Verification items for this drawing (mm, ordinates from the low corner). A direction names the side the tool comes from. Give positions to 0.01 mm unless a question says otherwise; leave off trailing zeros. Loops run counter-clockwise (first coordinate to the right, second up) from the corner with the lowest first, then second, coordinate; pieces in that order, holes last. Notation, with made-up numbers: M -33.5,17 L -1.5,17 A12 cw -1.5,31 Z; hole C 84,-2 d7. An arc over 180 degrees is marked long. Use a Markdown table: item, result.
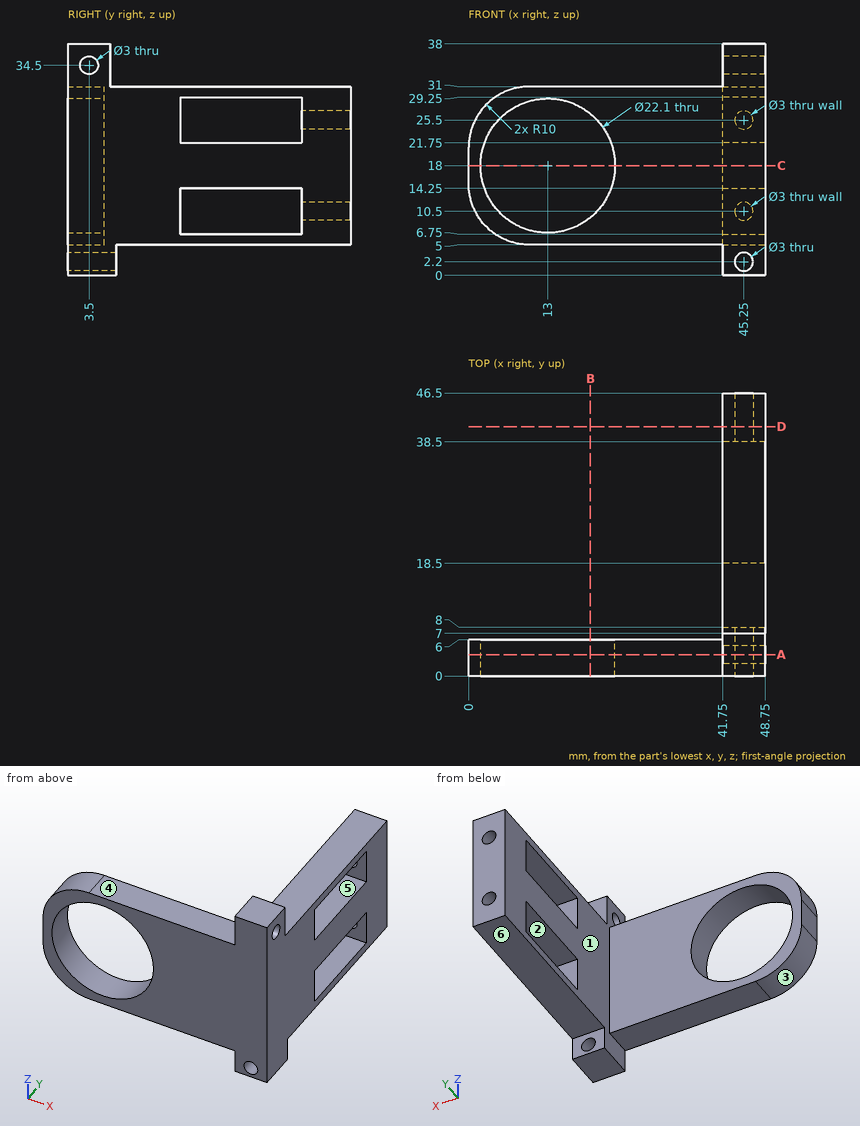
(1) Cross-section at C-C on z = 18. Record the cut outline in (x, y), then the cut area to 3 significant figures.
Results below:
| item | result |
|---|---|
| outline | M 0,0 L 1.95,0 L 1.95,6 L 0,6 Z; M 24.05,0 L 48.75,0 L 48.75,46.5 L 41.75,46.5 L 41.75,6 L 24.05,6 Z |
| area | 443 mm^2 |
(2) Cross-section at B-B on x = 20. Record the cut outline in (y, z).
Results below:
| item | result |
|---|---|
| outline | M 0,5 L 6,5 L 6,9.45 L 0,9.45 Z; M 0,26.55 L 6,26.55 L 6,31 L 0,31 Z |
(3) Set-up check for the marked faces 4, 5 and 6: record each of +Z, -Z, +X, -X, +Y, -Y from which the full face is reachable in a straight line by a thin tool's end or side.
Results below:
| item | result |
|---|---|
| face 4 | +Z, -X, +Y, -Y |
| face 5 | +X, -X |
| face 6 | -Z, +X, -X, +Y |
(4) Cross-section at D-D on y = 41. Record the cut outline in (x, z), then the cut area to 3 significant figures.
Results below:
| item | result |
|---|---|
| outline | M 41.75,5 L 48.75,5 L 48.75,31 L 41.75,31 Z; hole C 45.25,10.5 d3; hole C 45.25,25.5 d3 |
| area | 168 mm^2 |
(5) Material ranges on line 1 (Z direction, x = 13, y = 2.1); line 2 (Z direction, x = 45.25, y = 41.5); line 3 (X direction, y = 2, z = 2.2), recorded low to high.
Results below:
| item | result |
|---|---|
| line 1 | 5 to 6.95, 29.05 to 31 |
| line 2 | 5 to 9, 12 to 24, 27 to 31 |
| line 3 | 41.75 to 43.75, 46.75 to 48.75 |
(6) Gauge pin test, flat ends, axial feed: P1, Ø3.5, axis at x = 45, y = 31, coming from the +Z side; P2, Ø1.5, axis at x = 44, z = 1.5, coming from the +Y side; P3, Ø10, axis at x = 30.5, z = 6.5, coming from the +Y side. Record the tip position at first contact, or that the pin passes through.
Results below:
| item | result |
|---|---|
| P1 | z = 31 |
| P2 | y = 8 |
| P3 | y = 6 |
(7) Cross-section at A-A on y = 3.5. Record the cut outline in (x, z).
Results below:
| item | result |
|---|---|
| outline | M 0,15 A10 ccw 10,5 L 41.75,5 L 41.75,0 L 48.75,0 L 48.75,33 L 41.75,33 L 41.75,31 L 10,31 A10 ccw 0,21 Z; M 41.75,36 L 48.75,36 L 48.75,38 L 41.75,38 Z; hole C 13,18 d22.1; hole C 45.25,2.2 d3 |
(8) Draft check along Z on the marked faces 1, 2 and 3. Enter one of: +Z half, -Z half, draft (parallel to the pull), parting line (faces both ways), or undercut.
Results below:
| item | result |
|---|---|
| face 1 | draft |
| face 2 | undercut |
| face 3 | -Z half |
